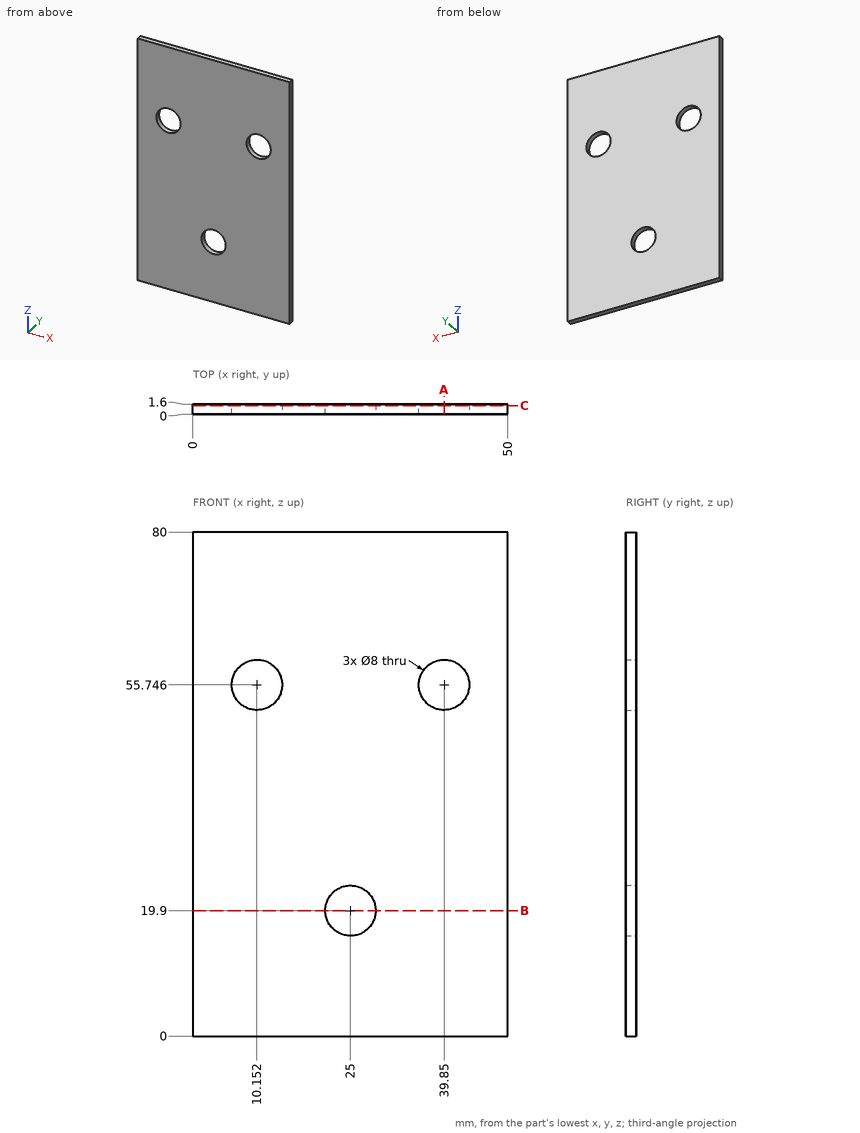
Job drawing, mm, ordinate dimensions from the low corner. One solid piece. Round coordinates to 2 decimals unless told otherwise and drop trailing zeros. Loops run counter-clockwise (first coordinate to the right, second up) from the corner with the lowest first, then second, coordinate; pieces in that order, holes last. Notation, with made-up numbers: (6, -36) -> (20, -36) arc R31 cw to (20, 2) -> close; hole circle Ø2 at (-1.5, 76). An arc over 180 degrees is marked (long way). Use a Markdown table: item, result.
1) Cut at C-C, the plane y = 1.35. List the corners of the cut face in (x, z).
The answers:
| item | result |
|---|---|
| outline | (0, 0) -> (50, 0) -> (50, 80) -> (0, 80) -> close; hole circle Ø8 at (10.15, 55.75); hole circle Ø8 at (25, 19.9); hole circle Ø8 at (39.85, 55.75) |
2) Probe line 1 (Z direction, x = 25, y = 1.3); line 2 (X direction, y = 0.6, z = 19.9); line 3 (X direction, y = 1.15, z = 53). List the from-to ranges inside material, lowest first. Write a range as [from, to].
The answers:
| item | result |
|---|---|
| line 1 | z = [0, 15.9], [23.9, 80] |
| line 2 | x = [0, 21], [29, 50] |
| line 3 | x = [0, 7.24], [13.06, 36.94], [42.76, 50] |
3) Cut at B-B, the plane z = 19.9. List the corners of the cut face in (x, y), and give its area (3 significant figures).
The answers:
| item | result |
|---|---|
| outline | (0, 0) -> (21, 0) -> (21, 1.6) -> (0, 1.6) -> close; (29, 0) -> (50, 0) -> (50, 1.6) -> (29, 1.6) -> close |
| area | 67.2 mm2 |
4) Cut at A-A, the plane x = 39.85. List the corners of the cut face in (y, z), and give its area (3 significant figures).
The answers:
| item | result |
|---|---|
| outline | (0, 0) -> (1.6, 0) -> (1.6, 51.75) -> (0, 51.75) -> close; (0, 59.75) -> (1.6, 59.75) -> (1.6, 80) -> (0, 80) -> close |
| area | 115 mm2 |
